Read the model definition and answer for the solid it produces. Units are mm, in the model's axes. A direction names the side the tool comes from. Give positions to 0.01 mm unless a question says otherwise; leave off trailing zeros. Loops run counter-clockwise (first coordinate to the right, second up) from the corner with the lowest first, then second, coordinate; pieces in that order, holes last. Notation, with made-up numbers: (67, 13.5) - (99, 13.5) arc R15 cw to (99, 27.5) - close; hole circle Ø8 at (89, -7). An arc over 180 degrees is marked (long way). Write item = value, one per line. Start each with the question number.
from build123d import *

# Parameters (mm, degrees)
EXTRUDE_1_DEPTH = 41.5


with BuildPart() as part:
    # 草图1 → 凸台-拉伸1 (new body)
    with BuildSketch(Plane.ZY):
        with BuildLine():
            Line((-247.135706549, 691.329742198), (233.685421601, 659.136990159))
            ThreePointArc((233.685421601, 659.136990159), (253.25995653, 648.399148569), (255.023393056, 626.142600064))
            Line((255.023393056, 626.142600064), (221.292164335, 521.502399447))
            ThreePointArc((221.292164335, 521.502399447), (212.760551455, 509.716531999), (198.925533748, 505.212381151))
            Line((198.925533748, 505.212381151), (-86.132619056, 505.212381151))
            ThreePointArc((-86.132619056, 505.212381151), (-94.324335579, 506.686356081), (-101.488444886, 510.923378563))
            Line((-101.488444886, 510.923378563), (-262.649988816, 650.041273838))
            ThreePointArc((-262.649988816, 650.041273838), (-269.292445055, 676.096205655), (-247.135706549, 691.329742198))
        make_face()
        with BuildLine():
            Line((-259.709511529, 653.447678589), (-98.547967599, 514.329783314))
            ThreePointArc((-98.547967599, 514.329783314), (-92.75570901, 510.904105562), (-86.132619056, 509.712381151))
            Line((-86.132619056, 509.712381151), (198.925533748, 509.712381151))
            ThreePointArc((198.925533748, 509.712381151), (210.111292745, 513.354035028), (217.00919252, 522.883034241))
            Line((217.00919252, 522.883034241), (250.816171993, 627.758227005))
            ThreePointArc((250.816171993, 627.758227005), (249.506743796, 645.91598122), (233.526965164, 654.637524387))
            Line((233.526965164, 654.637524387), (-247.294162986, 686.830276426))
            ThreePointArc((-247.294162986, 686.830276426), (-265.102438575, 674.453366381), (-259.709511529, 653.447678589))
        make_face(mode=Mode.SUBTRACT)
    extrude(amount=EXTRUDE_1_DEPTH)


solid = part.part
1. Consider line 1 along Y through (x, z) = (-30, -137.5); line 2 along Y through (x, z) = (-21.5, 109); line 3 along Z through (x, y) = (-26, 526). Determine where each line is inside the solid, lowest interval first. Write a range as [from, to].
2. A cutting plane is placed at A-A on x = -10. Give the vertices of the cut face in (y, z).
3. For a pull along Y with two mould halves and no side action, classify faces 1 (the flat face through (-20.46, 579.51, -180.94)), 2 (the flat face through (-20.46, 675.46, -10.09)), 3 (the flat face through (-20.46, 574.587, 233.676)) as released by +Y, released by -Y, zero draft, split by the parting line, or undercut.
4. A tool of negligible diameter and unlimited length cuts with its end or side. For faces 4 (the flat face through (0, 509, 14)), 5 (the cylindrical face through (-20.46, 510.937, -92.844)), from which of +Z, -Z, +X, -X, +Y, -Y can it reach the whole face along a straight path? Write none if from no direction.
5. A cutting plane is placed at C-C on y = 641.5. Give the vertices of the cut face in (x, z), and give its area (3 significant figures).
6. A cutting plane is placed at B-B on z = -19.5. Give the vertices of the cut face in (x, y), and give its area (3 significant figures).
7. Given P1, Ø6, axis at x = -9, y = 573.5, coming from the +Z side; P2, Ø12.5, axis at x = -25.5, z = 96, coming from the +Y side; P3, Ø4, axis at x = -10, y = 665, coming from the -Z side, each flat-ended and moving along its own axis, determine where each tip first touches the part or whether it passes through.
Reply:
q1.line_1 = [542.01, 547.95], [679.48, 683.99]
q1.line_2 = [505.21, 509.71], [662.98, 667.49]
q1.line_3 = [-118.95, -112.07], [218.01, 222.74]
q2.outline = (505.21, -86.13) arc R23.5 ccw to (510.92, -101.49) - (650.04, -262.65) arc R23.5 ccw to (691.33, -247.14) - (659.14, 233.69) arc R23.5 ccw to (626.14, 255.02) - (521.5, 221.29) arc R23.5 ccw to (505.21, 198.93) - close; hole (509.71, -86.13) arc R19 ccw to (514.33, -98.55) - (653.45, -259.71) arc R19 ccw to (686.83, -247.29) - (654.64, 233.53) arc R19 ccw to (627.76, 250.82) - (522.88, 217.01) arc R19 ccw to (509.71, 198.93) - close
q3.face_1 = released by -Y
q3.face_2 = released by +Y
q3.face_3 = undercut
q4.face_4 = +Z, -Z, +X, +Y, -Y
q4.face_5 = +X, -X
q5.outline = (-41.5, -252.76) - (0, -252.76) - (0, -245.87) - (-41.5, -245.87) - close; (-41.5, 251.6) - (0, 251.6) - (0, 256.28) - (-41.5, 256.28) - close
q5.area = 480 mm^2
q6.outline = (-41.5, 505.21) - (0, 505.21) - (0, 509.71) - (-41.5, 509.71) - close; (-41.5, 671.58) - (0, 671.58) - (0, 676.09) - (-41.5, 676.09) - close
q6.area = 374 mm^2
q7.P1 = 239.02
q7.P2 = 668.77
q7.P3 = -270.78
